Part model, mm, in its own coordinate system. Face numbers are marked on the shaded views. A direction names the side the tool comes from. Give positions to 0.01 mm unless a question says otherwise; leave off trailing zeros. Order: outer loops, then holes, each group sorted by start corner. A loop starts at its lowest first (then second) coordinate and runs counter-clockwise, first axis right, second up. Notation, with made-up numbers: (52, 74) -> (101, 74) arc R23 ccw to (101, 94) -> close; hole circle Ø5 at (55.25, -29.75). An arc over 180 degrees is marked (long way). Write item = value, one per line. Start each with the question number.
(1) Saw through at C-C, the plane z = 10. State how many separate pieces and enclosed holes the cut face has, then the cut area to 3 significant figures.
(2) Flat gauge pins, fed straight in: pin 1 (8 mm diameter, centred on x = 18.5, z = 8.5, fed in from +Y); pin 2 (5 mm diameter, centred on x = 14, z = 8, fed in from +Y). Where does each tip first touch, or does it go through?
(3) Two-plate mould, pull along X, no slides. Class the marked faces 6, 7 and 8: pulls with the +X half, pulls with the -X half, needs draft (parallel to the pull), parting line crosses it, or undercut.
(4) Saw through at D-D, the plane x = 4.5. List the corners of the cut face in (y, z), then the cut area to 3 significant figures.
(5) Which spindle directions (+Z, -Z, +X, -X, +Y, -Y) get a long thin tool onto all of the face, cutting with end or side? Do the marked faces 1, 2, 3, 4 and 5. Say none if no direction does.
(6) Saw through at B-B, the plane x = 14.25. List the corners of the cut face in (y, z).
(7) Probe line 1 along Z through (x, y) = (14.25, 7.2); line 2 along X through (y, z) = (19, 7.5); line 3 along Z through (x, y) = (24.85, 20). List the from-to ranges inside material, lowest first. Write a range as from..to.
(8) Saw through at A-A, the plane y = 16. List the corners of the cut face in (x, z).
from build123d import *

# Parameters (mm, degrees)
F1_DEPTH  = 20
F2_R      = 2.5
F3_DEPTH  = 30.001
F4_R      = 5
F5_DEPTH  = 6
F7_DEPTH  = 20
F8_SIZE   = 1
F9_R      = 2.65
F10_DEPTH = 28.501


with BuildPart() as f1:
    # F0 (on Top) → F1 (new body)
    with BuildSketch(Plane.XY):
        Polygon((0, 30), (0, 0), (28.5, 0), (28.5, 30), (24.5, 30), (24.5, 10), (4, 10), (4, 30), align=None)
    extrude(amount=F1_DEPTH)

    # F2 (on Front) → F3 (cut, through all)
    with BuildSketch(Plane.XZ):
        with Locations((14.25, 10)):
            Circle(F2_R)
    extrude(amount=-F3_DEPTH, mode=Mode.SUBTRACT)

    # F4 (on face) → F5 (cut)
    with BuildSketch(Plane(origin=(0, 10, 0), x_dir=(-1, 0, 0), z_dir=(0, 1, 0))):
        with Locations((-14.25, 10)):
            Circle(F4_R)
    extrude(amount=-F5_DEPTH, mode=Mode.SUBTRACT)

    # F6 (on Top) → F7 (join, through all)
    with BuildSketch(Plane.XY):
        Polygon((4, 24.5), (4, 15.5), (5, 16.5), (5, 23.5), align=None)
        Polygon((23.5, 16.5), (24.5, 15.5), (24.5, 24.5), (23.5, 23.5), align=None)
    extrude(amount=F7_DEPTH)

    # F8
    f8_edges = [f1.edges().sort_by_distance(p)[0] for p in [
        (5, 20, 20),
        (5, 20, 0),
        (23.5, 20, 20),
        (23.5, 20, 0),
    ]]
    chamfer(f8_edges, length=F8_SIZE)

    # F9 (on Right) → F10 (cut, through all)
    with BuildSketch(Plane.YZ):
        with Locations((20, 10)):
            Circle(F9_R)
    extrude(amount=F10_DEPTH, mode=Mode.SUBTRACT)


solid = f1.part
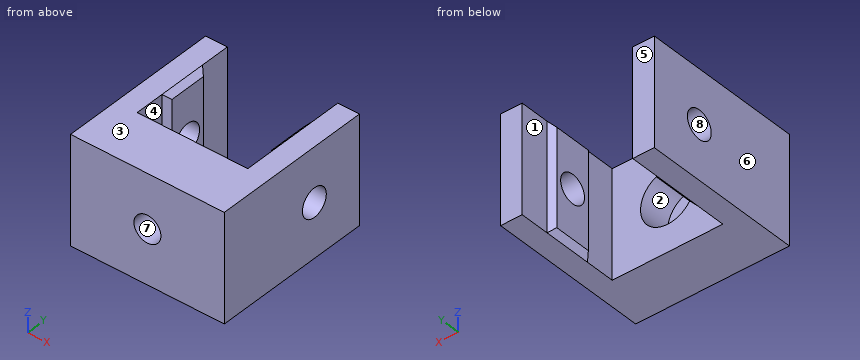
Results list:
q1.separate_pieces = 4
q1.enclosed_holes = 0
q1.area = 328 mm^2
q2.pin_1 = 10
q2.pin_2 = 4
q3.face_6 = pulls with the -X half
q3.face_7 = undercut
q3.face_8 = needs draft
q4.outline = (0, 0) -> (10, 0) -> (10, 20) -> (0, 20) -> close; (16, 0.5) -> (24, 0.5) -> (24, 19.5) -> (16, 19.5) -> close; hole circle Ø5.3 at (20, 10)
q4.area = 330 mm^2
q5.face_1 = +Z, -Z, +Y
q5.face_2 = +Y
q5.face_3 = +Z, +X, -X, +Y, -Y
q5.face_4 = +Z, -Z
q5.face_5 = +Z, -Z, +X, -X, +Y
q6.outline = (0, 0) -> (10, 0) -> (10, 5) -> (4, 5) -> (4, 7.5) -> (0, 7.5) -> close; (0, 12.5) -> (4, 12.5) -> (4, 15) -> (10, 15) -> (10, 20) -> (0, 20) -> close
q7.line_1 = 0..5, 15..20
q7.line_2 = 0..5, 23.5..28.5
q7.line_3 = 0..7.35, 12.65..20
q8.outline = (0, 0) -> (4, 0) -> (4.5, 0.5) -> (4.5, 19.5) -> (4, 20) -> (0, 20) -> close; (24, 0.5) -> (24.5, 0) -> (28.5, 0) -> (28.5, 20) -> (24.5, 20) -> (24, 19.5) -> close
